Geometry check sheet. Reference: the model listing, model coordinates, mm. Face numbers are marked on the shaded views. A direction names the side the tool comes from. Give positions to 0.01 mm unless a question says otherwise; leave off trailing zeros. Loops run counter-clockwise (first coordinate to the right, second up) from the corner with the lowest first, then second, coordinate; pieces in that order, holes last. Notation, with made-up numbers: (89.5, 20) -> (118.5, 20) arc R34 ccw to (118.5, 52) -> close; hole circle Ø2 at (30, 82). An arc over 180 degrees is marked (long way). Answer in a Markdown table with one row per item. Add a question column.
```python
from build123d import *

# Parameters (mm, degrees)
F1_W     = 130.1261633635
F1_H     = 82.6476961374
F1_W_2   = 112.0021492243
F1_H_2   = 63.2450655103
F2_DEPTH = 81.026
F3_W     = 57.0448189974
F3_H     = 46.4622946749
F4_DEPTH = 105.156
F5_R     = 11.4594947591
F6_DEPTH = 164.338


with BuildPart() as f2:
    # F1 (on face) → F2 (new body)
    with BuildSketch(Plane.XY):
        Rectangle(F1_W, F1_H)
        Rectangle(F1_W_2, F1_H_2, mode=Mode.SUBTRACT)
    extrude(amount=F2_DEPTH)

    # F3 (on face) → F4 (cut)
    with BuildSketch(Plane(origin=(0, 41.3238480687, 0), x_dir=(-1, 0, 0), z_dir=(0, 1, 0))):
        with Locations((0.1007858664, 57.7948526626)):
            Rectangle(F3_W, F3_H)
    extrude(amount=-F4_DEPTH, mode=Mode.SUBTRACT)

    # F5 (on face) → F6 (cut)
    with BuildSketch(Plane(origin=(-65.0630816817, 0, 0), x_dir=(0, -1, 0), z_dir=(-1, 0, 0))):
        with Locations((0, 42.6265746355)):
            Circle(F5_R)
    extrude(amount=-F6_DEPTH, mode=Mode.SUBTRACT)


solid = f2.part
```
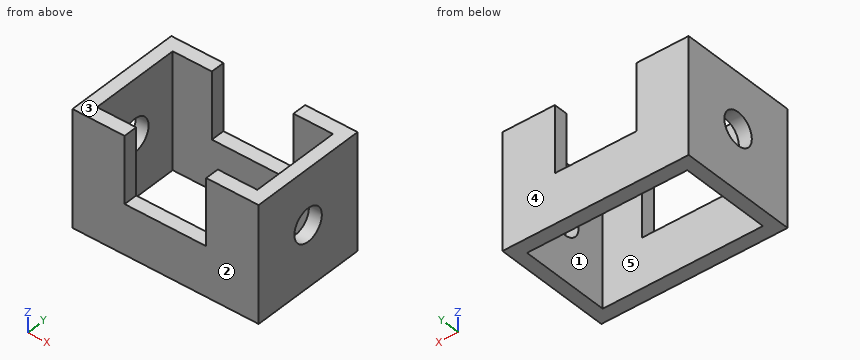
1. Sectioned sample at D-D (y = 0). Enter the section's corners in (x, z).
2. Release check for a two-part mould opening along Y. For the marked faces 1, 2 and 3 record: released by +Y, released by -Y, zero draft, split by the parting line, or undercut.
3. Material ranges on L1, parallel to Y at x = -50, z = 63.5; L2, parallel to Z at x = 62, y = 0; L3, parallel to X at y = -35, z = 70, recorded low to high. Write a range as from..to.
4. Sectioned sample at C-C (z = 73). Enter the section's corners in (x, y).
5. Gauge pin test, flat end, axial feed: pin 1 Ø5 at (x, y) = (10, 37.5) entering from +Z. Record the tip position at first contact, or that the pin passes through.
6. Sectioned sample at B-B (z = 24.5). Enter the section's corners in (x, y).
7. Access from +Z, -Z, +X, -X, +Y, -Y to the whole of each face (thin tool, end or side, straight path). Record for the marked faces 4 and 5.
8. Sectioned sample at A-A (x = -3). Enter the section's corners in (y, z).
Response:
| question | item | result |
|---|---|---|
| 1 | outline | (-65.06, 0) -> (-56, 0) -> (-56, 31.17) -> (-65.06, 31.17) -> close; (-65.06, 54.09) -> (-56, 54.09) -> (-56, 81.03) -> (-65.06, 81.03) -> close; (56, 0) -> (65.06, 0) -> (65.06, 31.17) -> (56, 31.17) -> close; (56, 54.09) -> (65.06, 54.09) -> (65.06, 81.03) -> (56, 81.03) -> close |
| 2 | face 1 | undercut |
| 2 | face 2 | released by -Y |
| 2 | face 3 | zero draft |
| 3 | L1 | y = -41.32..-31.62, 31.62..41.32 |
| 3 | L2 | z = 0..31.17, 54.09..81.03 |
| 3 | L3 | x = -65.06..-28.62, 28.42..65.06 |
| 4 | outline | (-65.06, -41.32) -> (-28.62, -41.32) -> (-28.62, -31.62) -> (-56, -31.62) -> (-56, 31.62) -> (-28.62, 31.62) -> (-28.62, 41.32) -> (-65.06, 41.32) -> close; (28.42, -41.32) -> (65.06, -41.32) -> (65.06, 41.32) -> (28.42, 41.32) -> (28.42, 31.62) -> (56, 31.62) -> (56, -31.62) -> (28.42, -31.62) -> close |
| 5 | pin 1 | stops at z = 34.56 |
| 6 | outline | (-65.06, -41.32) -> (65.06, -41.32) -> (65.06, 41.32) -> (-65.06, 41.32) -> close; hole (-56, -31.62) -> (56, -31.62) -> (56, 31.62) -> (-56, 31.62) -> close |
| 7 | face 4 | +Z, -Z, +X, -X, +Y |
| 7 | face 5 | +Z, -Z |
| 8 | outline | (-41.32, 0) -> (-31.62, 0) -> (-31.62, 34.56) -> (-41.32, 34.56) -> close; (31.62, 0) -> (41.32, 0) -> (41.32, 34.56) -> (31.62, 34.56) -> close |
